from build123d import *

# Parameters (mm, degrees)
SKETCH_1_R               = 10
EXTRUDE_1_DEPTH          = 20
SKETCH_2_R               = 4.5
CUT_EXTRUDE_1_DEPTH      = 20
CUT_EXTRUDE_2_DEPTH      = 86.562842403
CUT_EXTRUDE_2_DEPTH_BACK = 86.562842403


with BuildPart() as part:
    # 草图1 → 凸台-拉伸1 (new, symmetric)
    with BuildSketch(Plane.XY):
        with BuildLine():
            Line((0, -75), (18, -75))
            Line((18, -75), (18, -15))
            Line((18, -15), (15, 0))
            ThreePointArc((15, 0), (0, 15), (-15, 0))
            Line((-15, 0), (-18, -15))
            Line((-18, -15), (-18, -75))
            Line((-18, -75), (0, -75))
        make_face()
        Circle(SKETCH_1_R, mode=Mode.SUBTRACT)
    extrude(amount=EXTRUDE_1_DEPTH, both=True)

    # 草图2 → 切除-拉伸1 (cut, symmetric)
    with BuildSketch(Plane(origin=(0, 0, 0), x_dir=(0, 0, -1), z_dir=(1, 0, 0))):
        with Locations((0, -45)):
            Circle(SKETCH_2_R)
        with Locations((0, -25)):
            Circle(SKETCH_2_R)
        with Locations((0, -65)):
            Circle(SKETCH_2_R)
    extrude(amount=CUT_EXTRUDE_1_DEPTH, both=True, mode=Mode.SUBTRACT)

    # 草图7 → 切除-拉伸2 (cut, two sides: drawn at the far end of the back side and taken through both)
    with BuildSketch(Plane(origin=(18, 0, 0), x_dir=(0, 0, -1), z_dir=(1, 0, 0)).offset(-CUT_EXTRUDE_2_DEPTH_BACK)):
        with BuildLine():
            Line((-10, -65), (-20, -35))
            Line((-20, -35), (-20, -75))
            Line((-20, -75), (0, -75))
            ThreePointArc((0, -75), (-7.071067812, -72.071067812), (-10, -65))
        make_face()
        with BuildLine():
            ThreePointArc((10, -65), (7.071067812, -72.071067812), (0, -75))
            Line((0, -75), (20, -75))
            Line((20, -75), (20, -35))
            Line((20, -35), (10, -65))
        make_face()
    extrude(amount=CUT_EXTRUDE_2_DEPTH + CUT_EXTRUDE_2_DEPTH_BACK, mode=Mode.SUBTRACT)


solid = part.part
Design review of the part built by this model. Coordinates are the model's own, in mm. Round coordinates to 2 decimals unless told otherwise and drop trailing zeros. Order: outer loops, then holes, each group sorted by start corner. A loop starts at its lowest first (then second) coordinate and runs counter-clockwise, first axis right, second up. Notation, with made-up numbers: M 79,39 L 122,39 A13 cw 122,52 Z; hole C -5.75,60.5 d2. An arc over 180 degrees is marked long. Answer as CSV lines item,"result". Start each with the question number.
1) Add section C-C (y = -45). Give the boundary of the cut face in (x, z).
2) The part is to be moulded in two halves that separate along X. For faces 1 (the face through (0, -50, -15)), 2 (the face through (-18, -38, 0)), 3 (the face through (-2.17, -9.76, -0.28)), 4 (the face through (16.52, -7.6, 0.28)), say which applies: +X half, -X half, draft (parallel to the pull), parting line (faces both ways), or undercut.
3) For pin 1 Ø4 at (x, y) = (-3.5, -43) entering from -Z; pin 2 Ø8 at (y, z) = (-65, 0) entering from -X; pin 3 Ø4 at (x, z) = (-3, -4) entering from -Y; pin 4 Ø8 at (x, y) = (-1.5, -41.5) entering from -Z, all flat-tipped, find the tip position at first contact; note any pin that passes through.
4) Wall thickness on line 1 along Y through (x, z) = (9, 4); line 2 along Y through (x, z) = (7, 2.5); line 3 along Y through (x, z) = (12, -1): over which ranges is each line inside the solid? List them lowest first. Write a range as [from, to].
5) Add section D-D (x = -12). Give the boundary of the cut face in (y, z).
6) Add section A-A (z = -14.5). Give the boundary of the cut face in (x, y), then the cut area to 3 significant figures.
7) Add section B-B (x = -7.5). Give the boundary of the cut face in (y, z), then the cut area to 3 significant figures.
Resolved:
1,outline,"M -18,-16.67 L 18,-16.67 L 18,-4.5 L -18,-4.5 Z; M -18,4.5 L 18,4.5 L 18,16.67 L -18,16.67 Z"
2,face 1,"draft"
2,face 2,"-X half"
2,face 3,"undercut"
2,face 4,"+X half"
3,pin 1,"z = -18"
3,pin 2,"through"
3,pin 3,"y = -74.8"
3,pin 4,"z = -19.17"
4,line 1,"[-74.17, -67.06], [-62.94, -47.06], [-42.94, -27.06], [-22.94, -4.36], [4.36, 12]"
4,line 2,"[-74.68, -68.74], [-61.26, -48.74], [-41.26, -28.74], [-21.26, -7.14], [7.14, 13.27]"
4,line 3,"[-74.95, -69.39], [-60.61, -49.39], [-40.61, -29.39], [-20.61, 9]"
5,outline,"M -65,-10 L -35,-20 L 9,-20 L 9,20 L -35,20 L -65,10 A10 ccw Z; hole C -65,0 d9; hole C -45,0 d9; hole C -25,0 d9"
6,outline,"M -18,-51.5 L 18,-51.5 L 18,-15 L 15,0 A15 ccw -15,0 L -18,-15 Z; hole C 0,0 d20"
6,area,"1,850 mm^2"
7,outline,"M -65,-10 L -35,-20 L -6.61,-20 L -6.61,20 L -35,20 L -65,10 A10 ccw Z; M 6.61,-20 L 12.99,-20 L 12.99,20 L 6.61,20 Z; hole C -65,0 d9; hole C -45,0 d9; hole C -25,0 d9"
7,area,"2,260 mm^2"
